The model under review builds one solid part; all positions refer to its coordinate system, in mm. A direction names the side the tool comes from. Give positions to 0.01 mm unless a question says otherwise; leave off trailing zeros. Order: outer loops, then holes, each group sorted by start corner. A loop starts at its lowest first (then second) coordinate and runs counter-clockwise, first axis right, second up. Notation, with made-up numbers: (-32.5, 28) - (3.5, 28) arc R18 cw to (3.5, 49) - close; hole circle Ø10 at (19.5, 24). An arc over 180 degrees is marked (long way). Use CSV: the item, a comma, the result in double quotes. Start each with the question number.
1. Machinability: for faces 1 (the flat face through (1, 1, 0)), 2 (the flat face through (-4, -13, 10)), 3 (the flat face through (3, 0, 5)), which of the approach directions +Z, -Z, +X, -X, +Y, -Y give a long, thin tool a straight path to every point of the face, cutting with its end or side? Answer none if there is none.
2. Take a section at C-C, the plane z = 5.75. State the section outline as (x, y) points.
3. Draft analysis for pull direction Y (two halves, no side actions). For faces 4 (the cylindrical face through (1.94, -0.61, -5.07)), 5 (the cylindrical face through (-2.17, 9.76, -2.96)), 6 (the flat face through (7.3, -7.3, 0)), state which applies: released by +Y, released by -Y, zero draft, split by the parting line, or undercut.
4. To check wall thickness, follow line 1 (Y direction, x = 0, z = 9); line 2 (Y direction, x = 0, z = 2.75); line 3 (Z direction, x = 14, y = -0.5). State the ranges of each line that lie inside material, in increasing order. Write a range as [from, to].
5. Take a section at A-A, the plane x = 0. State the section outline as (y, z) points.
6. Take a section at D-D, the plane y = -12. State the section outline as (x, z) points.
7. For pin 1 (1 mm diameter, centred on x = 7.5, z = 5, fed in from +Y); pin 2 (2.5 mm diameter, centred on x = 0, y = 0, fed in from -Z); pin 3 (2 mm diameter, centred on x = 5, y = 6.5, fed in from -Z), all flat-tipped, find the tip position at first contact; note any pin that passes through.
```python
from build123d import *

# Parameters (mm, degrees)
CYLINDER_R      = 17
CYLINDER_DEPTH  = 10
SKETCH_R        = 13
POCKET_DEPTH    = 5
SKETCH001_R     = 10
PAD_DEPTH       = 10
FILLET_R        = 4
SKETCH002_R     = 2.03183
POCKET001_DEPTH = 10
SKETCH003_R     = 1.012126
POCKET002_DEPTH = 15.001


with BuildPart() as part:
    # Cylinder → Cylinder (new body)
    with BuildSketch(Plane.XY):
        Circle(CYLINDER_R)
    extrude(amount=CYLINDER_DEPTH)

    # Sketch → Pocket (cut)
    with BuildSketch(Plane.XY.offset(10)):
        Circle(SKETCH_R)
    extrude(amount=-POCKET_DEPTH, mode=Mode.SUBTRACT)

    # Sketch001 → Pad (new body)
    with BuildSketch(Plane(origin=(0, 0, 0), x_dir=(1, 0, 0), z_dir=(0, 0, -1))):
        Circle(SKETCH001_R)
    extrude(amount=PAD_DEPTH)

    # Fillet
    fillet_edges = [part.edges().sort_by_distance(p)[0] for p in [
        (-10, 0, -10),
    ]]
    fillet(fillet_edges, radius=FILLET_R)

    # Sketch002 → Pocket001 (cut)
    with BuildSketch(Plane(origin=(0, 0, -10), x_dir=(1, 0, 0), z_dir=(0, 0, -1))):
        Circle(SKETCH002_R)
    extrude(amount=-POCKET001_DEPTH, mode=Mode.SUBTRACT)

    # Sketch003 → Pocket002 (cut, through all)
    with BuildSketch(Plane.XY.offset(5)):
        Circle(SKETCH003_R)
    extrude(amount=-POCKET002_DEPTH, mode=Mode.SUBTRACT)


solid = part.part
```
Determined:
1,face 1,"-Z"
1,face 2,"+Z, +X, -X, +Y, -Y"
1,face 3,"+Z"
2,outline,"circle Ø34 at (0, 0); hole circle Ø26 at (0, 0)"
3,face 4,"undercut"
3,face 5,"split by the parting line"
3,face 6,"zero draft"
4,line 1,"y = [-17, -13], [13, 17]"
4,line 2,"y = [-17, -1.01], [1.01, 17]"
4,line 3,"z = [0, 10]"
5,outline,"(-17, 0) - (-10, 0) - (-10, -6) arc R4 ccw to (-6, -10) - (-2.03, -10) - (-2.03, 0) - (-1.01, 0) - (-1.01, 5) - (-13, 5) - (-13, 10) - (-17, 10) - close; (1.01, 0) - (2.03, 0) - (2.03, -10) - (6, -10) arc R4 ccw to (10, -6) - (10, 0) - (17, 0) - (17, 10) - (13, 10) - (13, 5) - (1.01, 5) - close"
6,outline,"(-12.04, 0) - (12.04, 0) - (12.04, 10) - (5, 10) - (5, 5) - (-5, 5) - (-5, 10) - (-12.04, 10) - close"
7,pin 1,"stops at y = 15.49"
7,pin 2,"stops at z = 0"
7,pin 3,"stops at z = -9.82"
